Autodesk Inventor part; units mm, degrees
ref_plane "YZ Plane" through (0, 0, 0) normal (1, 0, 0) x (0, 1, 0)
ref_plane "XZ Plane" through (0, 0, 0) normal (0, 1, 0) x (-1, 0, 0)
ref_plane "XY Plane" through (0, 0, 0) normal (0, 0, 1) x (1, 0, 0)
sketch "Sketch1" plane through (0, 0, 0) normal (0, 0, 1) x (1, 0, 0)
  line L0 (0, 0) -> (10, 0)
  line L1 (0, 0) -> (-10, 0)
  line L2 (-10, 0) -> (-10, -6.5)
  line L3 (10, 0) -> (10, -6.5)
  line L4 (-10, 0) -> (10, 0)
  line L5 (-10, -20) -> (10, -20)
  line L6 (-10, -6.5) -> (-10, -5)
  line L7 (-6, -5) -> (6, -5)
  line L8 (-6, -15) -> (6, -15)
  line L9 (6, -5) -> (6, -15)
  line L10 (-6, -5) -> (-6, -15)
  line L11 (-10, 0) -> (-10, -6.5)
  line L12 (-10, -13.5) -> (-10, -20)
  line L13 (10, -20) -> (10, -13.5)
  line L14 (10, -6.5) -> (10, 0)
  circle A0 centre (10, -10) radius 1.5
  arc A1 (10, -13.5) -> (10, -6.5) centre (10, -10) ccw
  circle A2 centre (-10, -10) radius 1.5
  arc A3 (-10, -6.5) -> (-10, -13.5) centre (-10, -10) ccw
  dimension "d0" = 10
  dimension "d1" = 10
  dimension "d2" = 20
  dimension "d7" = 3
  dimension "d8" = 7
  dimension "d9" = 3
  dimension "d10" = 7
extrude "Extrusion1" add sketch "Sketch1" along normal blind 2
thread "Thread2"
thread "Thread3"
sketch "Sketch6" plane through (0, 0, 2) normal (0, 0, 1) x (1, 0, 0)
  line L0 (10, 0) -> (-10, 0)
  line L1 (-5, 0) -> (-5, 20)
  line L2 (-5, 0) -> (15, 0) construction
  line L3 (-5, 20) -> (5, 20)
  line L4 (5, 20) -> (5, 0)
  arc A0 (-10, -6.5) -> (-10, -13.5) centre (-10, -10) ccw
  arc A1 (10, -13.5) -> (10, -6.5) centre (10, -10) ccw
  line L5 (0, 20) -> (0, 9.84)
  circle A2 centre (0, 14.92) radius 2.125
  line L6 (0, 0) -> (0, 10.16)
  circle A3 centre (0, 5.08) radius 2.125
  line L7 (-2.125, 14.92) -> (-2.125, 5.08)
  line L8 (2.125, 14.92) -> (2.125, 5.08)
  line L9 (-13.5, -10) -> (13.5, -10)
  line L10 (10, -20) -> (-10, -20)
  line L11 (-5, -20) -> (-5, -40)
  line L12 (-5, -40) -> (5, -40)
  line L13 (5, -40) -> (5, -20)
  line L14 (0, -40) -> (0, -29.84)
  circle A4 centre (0, -34.92) radius 2.125
  line L15 (0, -20) -> (0, -30.16)
  circle A5 centre (0, -25.08) radius 2.125
  line L16 (-2.125, -34.92) -> (-2.125, -25.08)
  line L17 (2.125, -34.92) -> (2.125, -25.08)
  dimension "d45" = 20
  dimension "d47" = 10
  dimension "d52" = 10.16
  dimension "d53" = 4.25
  dimension "d54" = 10.16
  dimension "d55" = 4.25
extrude "Extrusion7" add sketch "Sketch6" against normal blind 2 contours L0 L6 A3 L8 A2 L5 L3 L4 | L0 L1 L3 L5 A2 L7 A3 L6 | L13 L12 L14 A4 L17 A5 L15 L10 | L15 A5 L16 A4 L14 L12 L11 L10
fillet "Fillet2" radius 5 4 edges at (5, -40, 1) (-5, -40, 1) (5, 20, 1) (-5, 20, 1)
properties part number "Time of Flight Attachment"
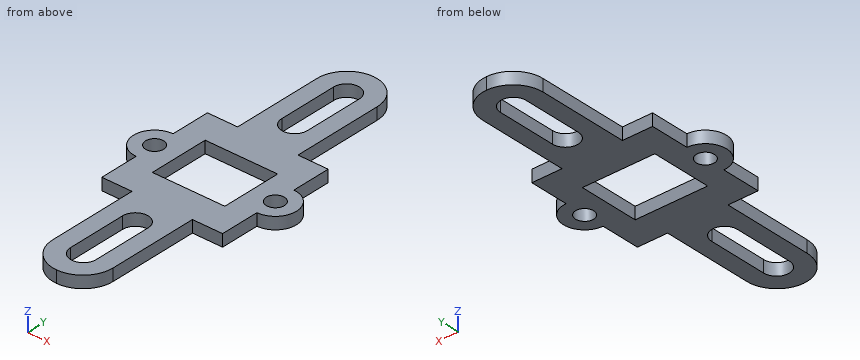
Source: CAD feature listing. Evaluate the final solid. Frame: model axes, mm. Give positions to 0.01 mm unless a question says otherwise; leave off trailing zeros. Order: outer loops, then holes, each group sorted by start corner. A loop starts at its lowest first (then second) coordinate and runs counter-clockwise, first axis right, second up. Notation, with made-up numbers: (-22, 88.25) -> (5, 88.25) arc R19 cw to (5, 122.25) -> close; hole circle Ø6 at (14, 1.5). An arc over 180 degrees is marked (long way). Use a Markdown table: item, result.
Q1. Section C-C (x = 3.75). Return the cut outline in (y, z).
A:
| item | result |
|---|---|
| outline | (-38.31, 0) -> (-15, 0) -> (-15, 2) -> (-38.31, 2) -> close; (-5, 0) -> (18.31, 0) -> (18.31, 2) -> (-5, 2) -> close |
Q2. Material intervals for line 1 (X direction, y = 8.5, z = 0.85) (3 decimals); line 2 (X direction, y = -2.5, z = 0.1); line 3 (Y direction, x = -0.75, z = 0.6), sorted ascending. Write a range as [from, to].
A:
| item | result |
|---|---|
| line 1 | [-5, -2.125], [2.125, 5] |
| line 2 | [-10, 10] |
| line 3 | [-39.94, -36.91], [-23.09, -15], [-5, 3.09], [16.91, 19.94] |
Q3. Section A-A (y = -26). Return the cut outline in (x, z) (3 decimals), and give its area (3 significant figures).
A:
| item | result |
|---|---|
| outline | (-5, 0) -> (-2.125, 0) -> (-2.125, 2) -> (-5, 2) -> close; (2.125, 0) -> (5, 0) -> (5, 2) -> (2.125, 2) -> close |
| area | 11.5 mm^2 |
Q4. First-contact query: P1, Ø1, axis at y = -30, z = 1.5, coming from the -X side; P2, Ø1, axis at x = 7, z = 1.5, coming from the +Y side; P3, Ø0.6, axis at y = -16.5, z = 0.5, coming from the +X side; P4, Ø5, axis at x = 7, y = 8, coming from the -Z side. Flat tips, straight axial feed; report the tip coordinate or a pass-through.
A:
| item | result |
|---|---|
| P1 | x = -5 |
| P2 | y = 0 |
| P3 | x = 10 |
| P4 | z = 0 |
Q5. Section D-D (y = -19). Return the cut outline in (x, z).
A:
| item | result |
|---|---|
| outline | (-10, 0) -> (10, 0) -> (10, 2) -> (-10, 2) -> close |
Q6. Section B-B (z = 1.6). State how many separate pieces and enclosed holes the cut face has, and give its area (3 significant figures).
A:
| item | result |
|---|---|
| separate pieces | 1 |
| enclosed holes | 5 |
| area | 571 mm^2 |
